```python
from build123d import *

# Parameters (mm, degrees)
F0_R     = 1.375
F0_R_2   = 4.5
F0_W     = 40
F0_H     = 10
F0_W_2   = 10
F0_H_2   = 35
F0_W_3   = 15
F0_H_3   = 2
F0_W_4   = 2
F0_W_5   = 5.5
F0_H_4   = 11.5
F0_R_3   = 1
F1_DEPTH = 3


# Not quite as in the source:
# - a feature names something its author has since deleted; it is built from what else it names


with BuildPart() as f1:
    # F0 (on Top) → F1 (new body)
    with BuildSketch(Plane.XY):
        with BuildLine():
            Line((25, 96.5), (-25, 96.5))
            ThreePointArc((-25, 96.5), (-32.0710678119, 93.5710678119), (-35, 86.5))
            Line((-35, 86.5), (-35, -86.5))
            ThreePointArc((-35, -86.5), (-32.0710678119, -93.5710678119), (-25, -96.5))
            Line((-25, -96.5), (25, -96.5))
            ThreePointArc((25, -96.5), (32.0710678119, -93.5710678119), (35, -86.5))
            Line((35, -86.5), (35, 86.5))
            ThreePointArc((35, 86.5), (32.0710678119, 93.5710678119), (25, 96.5))
        make_face()
        Polygon((-29, -86.5), (-29, -78), (-29, -55), (-29, -46.5), (-25.5, -46.5), (-25.5, -55), (-18.5, -55), (-13, -55), (-10.5, -55), (-10.5, -66.5), (-10.5, -78), (-10.5, -86.5), (-25.5, -86.5), align=None, mode=Mode.SUBTRACT)
        with Locations((-24.5, -8.5)):
            Circle(F0_R, mode=Mode.SUBTRACT)
        Polygon((10.5, -78), (10.5, -66.5), (10.5, -55), (13, -55), (18.5, -55), (24.5, -55), (25.5, -55), (25.5, -46.5), (29, -46.5), (29, -55), (29, -78), (29, -86.5), (25.5, -86.5), (10.5, -86.5), align=None, mode=Mode.SUBTRACT)
        with BuildLine():
            ThreePointArc((25.875, -8.5), (25.4722718241, -9.4722718241), (24.5, -9.875))
            ThreePointArc((24.5, -9.875), (23.5277281759, -7.5277281759), (25.875, -8.5))
        make_face(mode=Mode.SUBTRACT)
        with BuildLine():
            ThreePointArc((26, -30), (25.5980762114, -31.5), (24.5, -32.5980762114))
            ThreePointArc((24.5, -32.5980762114), (23.1822131445, -32.9944612821), (21.8260869565, -32.7607839768))
            ThreePointArc((21.8260869565, -32.7607839768), (0, -52), (-21.8260869565, -32.7607839768))
            ThreePointArc((-21.8260869565, -32.7607839768), (-26, -30), (-21.8260869565, -27.2392160232))
            ThreePointArc((-21.8260869565, -27.2392160232), (-16.3398685927, -15.268785034), (-5, -8.5757147144))
            Line((-5, -8.5757147144), (-5, -5.5))
            Line((-5, -5.5), (-14, -5.5))
            Line((-14, -5.5), (-14, -8.5))
            ThreePointArc((-14, -8.5), (-17, -11.5), (-20, -8.5))
            Line((-20, -8.5), (-20, -5.5))
            Line((-20, -5.5), (-30, -5.5))
            Line((-30, -5.5), (-32, -5.5))
            Line((-32, -5.5), (-32, 6.5))
            Line((-32, 6.5), (-32, 41.5))
            Line((-32, 41.5), (-32, 53.5))
            Line((-32, 53.5), (-30, 53.5))
            Line((-30, 53.5), (-30, 56.5))
            ThreePointArc((-30, 56.5), (-27, 59.5), (-24, 56.5))
            Line((-24, 56.5), (-24, 53.5))
            Line((-24, 53.5), (-20, 53.5))
            Line((-20, 53.5), (20, 53.5))
            Line((20, 53.5), (32, 53.5))
            Line((32, 53.5), (32, 41.5))
            Line((32, 41.5), (32, 6.5))
            Line((32, 6.5), (32, -5.5))
            Line((32, -5.5), (20, -5.5))
            Line((20, -5.5), (5, -5.5))
            Line((5, -5.5), (5, -8.5757147144))
            ThreePointArc((5, -8.5757147144), (16.3398685927, -15.268785034), (21.8260869565, -27.2392160232))
            ThreePointArc((21.8260869565, -27.2392160232), (23.1822131445, -27.0055387179), (24.5, -27.4019237886))
            ThreePointArc((24.5, -27.4019237886), (25.5980762114, -28.5), (26, -30))
        make_face(mode=Mode.SUBTRACT)
        with Locations((0, 81.5)):
            Circle(F0_R_2, mode=Mode.SUBTRACT)
        Polygon((5, 20), (5, 6.5), (20, 6.5), (20, 41.5), (-20, 41.5), (-20, 6.5), (-5, 6.5), (-5, 20), align=None)
        with BuildLine():
            ThreePointArc((-20, -30), (0, -50), (20, -30))
            ThreePointArc((20, -30), (15.8113883008, -17.7525512861), (5, -10.635083269))
            Line((5, -10.635083269), (5, -20))
            Line((5, -20), (-5, -20))
            Line((-5, -20), (-5, -10.635083269))
            ThreePointArc((-5, -10.635083269), (-15.8113883008, -17.7525512861), (-20, -30))
        make_face()
        with Locations((0, 46.5)):
            Rectangle(F0_W, F0_H)
        with Locations((-25, 24)):
            Rectangle(F0_W_2, F0_H_2)
        with Locations((25, 24)):
            Rectangle(F0_W_2, F0_H_2)
        Polygon((-29, -55), (-29, -78), (-25.5, -78), (-18.5, -78), (-18.5, -66.5), (-18.5, -55), (-25.5, -55), align=None)
        with Locations((-24.5, -66.5)):
            Circle(F0_R, mode=Mode.SUBTRACT)
        with BuildLine():
            Line((23.125, -66.5), (18.5, -66.5))
            Line((18.5, -66.5), (18.5, -78))
            Line((18.5, -78), (25.5, -78))
            Line((25.5, -78), (29, -78))
            Line((29, -78), (29, -55))
            Line((29, -55), (25.5, -55))
            Line((25.5, -55), (24.5, -55))
            Line((24.5, -55), (24.5, -65.125))
            ThreePointArc((24.5, -65.125), (25.4722718241, -65.5277281759), (25.875, -66.5))
            ThreePointArc((25.875, -66.5), (24.5, -67.875), (23.125, -66.5))
        make_face()
        with Locations((-12.5, 1.5)):
            Rectangle(F0_W_3, F0_H)
        with Locations((12.5, 1.5)):
            Rectangle(F0_W_3, F0_H)
        Polygon((-18.5, -78), (-25.5, -78), (-25.5, -86.5), (-10.5, -86.5), (-10.5, -78), (-13, -78), align=None)
        Polygon((13, -78), (10.5, -78), (10.5, -86.5), (25.5, -86.5), (25.5, -78), (18.5, -78), align=None)
        with BuildLine():
            ThreePointArc((-21.8260869565, -32.7607839768), (0, -52), (21.8260869565, -32.7607839768))
            ThreePointArc((21.8260869565, -32.7607839768), (20.4978270313, -31.6550318531), (20, -30))
            ThreePointArc((20, -30), (0, -50), (-20, -30))
            ThreePointArc((-20, -30), (-20.4978270313, -31.6550318531), (-21.8260869565, -32.7607839768))
        make_face()
        with Locations((25, 46.5)):
            Rectangle(F0_W_2, F0_H)
        with Locations((-25, 46.5)):
            Rectangle(F0_W_2, F0_H)
        with Locations((-25, 1.5)):
            Rectangle(F0_W_2, F0_H)
        with Locations((25, 1.5)):
            Rectangle(F0_W_2, F0_H)
        with Locations((0, 52.5)):
            Rectangle(F0_W, F0_H_3)
        with Locations((31, 24)):
            Rectangle(F0_W_4, F0_H_2)
        with Locations((-31, 24)):
            Rectangle(F0_W_4, F0_H_2)
        with BuildLine():
            Line((18.5, -55), (18.5, -66.5))
            Line((18.5, -66.5), (23.125, -66.5))
            ThreePointArc((23.125, -66.5), (23.5277281759, -65.5277281759), (24.5, -65.125))
            Line((24.5, -65.125), (24.5, -55))
            Line((24.5, -55), (18.5, -55))
        make_face()
        with Locations((-15.75, -72.25)):
            Rectangle(F0_W_5, F0_H_4)
        with Locations((-15.75, -60.75)):
            Rectangle(F0_W_5, F0_H_4)
        with Locations((15.75, -72.25)):
            Rectangle(F0_W_5, F0_H_4)
        with Locations((15.75, -60.75)):
            Rectangle(F0_W_5, F0_H_4)
        with BuildLine():
            ThreePointArc((-5, -8.5757147144), (-16.3398685927, -15.268785034), (-21.8260869565, -27.2392160232))
            ThreePointArc((-21.8260869565, -27.2392160232), (-20.4978270313, -28.3449681469), (-20, -30))
            ThreePointArc((-20, -30), (-15.8113883008, -17.7525512861), (-5, -10.635083269))
            Line((-5, -10.635083269), (-5, -8.5757147144))
        make_face()
        with BuildLine():
            ThreePointArc((20, -30), (20.4978270313, -28.3449681469), (21.8260869565, -27.2392160232))
            ThreePointArc((21.8260869565, -27.2392160232), (16.3398685927, -15.268785034), (5, -8.5757147144))
            Line((5, -8.5757147144), (5, -10.635083269))
            ThreePointArc((5, -10.635083269), (15.8113883008, -17.7525512861), (20, -30))
        make_face()
        Polygon((30, 41.5), (32, 41.5), (32, 53.5), (20, 53.5), (20, 51.5), (30, 51.5), align=None)
        Polygon((20, -3.5), (20, -5.5), (32, -5.5), (32, 6.5), (30, 6.5), (30, -3.5), align=None)
        Polygon((-14, -5.5), (-5, -5.5), (-5, -3.5), (-20, -3.5), (-20, -5.5), (-17, -5.5), align=None)
        with Locations((12.5, -4.5)):
            Rectangle(F0_W_3, F0_H_3)
        with BuildLine():
            ThreePointArc((-30, 56.5), (-29.1213203519, 54.3786796648), (-27.0000000236, 53.5))
            ThreePointArc((-27.0000000236, 53.5), (-24.8786796648, 54.3786796481), (-24, 56.5))
            ThreePointArc((-24, 56.5), (-27, 59.5), (-30, 56.5))
        make_face()
        with Locations((-27, 56.5)):
            Circle(F0_R_3, mode=Mode.SUBTRACT)
        with BuildLine():
            ThreePointArc((-14, -8.5), (-14.8786796564, -6.3786796564), (-17, -5.5))
            ThreePointArc((-17, -5.5), (-19.1213203436, -6.3786796564), (-20, -8.5))
            ThreePointArc((-20, -8.5), (-17, -11.5), (-14, -8.5))
        make_face()
        with Locations((-17, -8.5)):
            Circle(F0_R_3, mode=Mode.SUBTRACT)
        Polygon((-32, 41.5), (-30, 41.5), (-30, 51.5), (-30, 53.5), (-32, 53.5), align=None)
        Polygon((-30, -5.5), (-30, -3.5), (-30, 6.5), (-32, 6.5), (-32, -5.5), align=None)
        with BuildLine():
            ThreePointArc((-21.8260869565, -27.2392160232), (-26, -30), (-21.8260869565, -32.7607839768))
            ThreePointArc((-21.8260869565, -32.7607839768), (-21.9564786913, -31.3831281496), (-22, -30))
            ThreePointArc((-22, -30), (-21.9564786913, -28.6168718504), (-21.8260869565, -27.2392160232))
        make_face()
        with Locations((-23, -30)):
            Circle(F0_R_3, mode=Mode.SUBTRACT)
        Polygon((-30, 51.5), (-20, 51.5), (-20, 53.5), (-24, 53.5), (-27.0000000236, 53.5), (-30, 53.5), align=None)
        with Locations((-25, -4.5)):
            Rectangle(F0_W_2, F0_H_3)
        with BuildLine():
            ThreePointArc((21.8260869565, -32.7607839768), (23.1822131445, -32.9944612821), (24.5, -32.5980762114))
            Line((24.5, -32.5980762114), (24.5, -27.4019237886))
            ThreePointArc((24.5, -27.4019237886), (23.1822131445, -27.0055387179), (21.8260869565, -27.2392160232))
            ThreePointArc((21.8260869565, -27.2392160232), (21.9564786913, -28.6168718504), (22, -30))
            ThreePointArc((22, -30), (21.9564786913, -31.3831281496), (21.8260869565, -32.7607839768))
        make_face()
        with BuildLine():
            ThreePointArc((24, -30), (23, -31), (22, -30))
            ThreePointArc((22, -30), (23, -29), (24, -30))
        make_face(mode=Mode.SUBTRACT)
        with BuildLine():
            ThreePointArc((-22, -30), (-21.9564786913, -31.3831281496), (-21.8260869565, -32.7607839768))
            ThreePointArc((-21.8260869565, -32.7607839768), (-20.4978270313, -31.6550318531), (-20, -30))
            ThreePointArc((-20, -30), (-20.4978270313, -28.3449681469), (-21.8260869565, -27.2392160232))
            ThreePointArc((-21.8260869565, -27.2392160232), (-21.9564786913, -28.6168718504), (-22, -30))
        make_face()
        with BuildLine():
            ThreePointArc((20, -30), (20.4978270313, -31.6550318531), (21.8260869565, -32.7607839768))
            ThreePointArc((21.8260869565, -32.7607839768), (21.9564786913, -31.3831281496), (22, -30))
            ThreePointArc((22, -30), (21.9564786913, -28.6168718504), (21.8260869565, -27.2392160232))
            ThreePointArc((21.8260869565, -27.2392160232), (20.4978270313, -28.3449681469), (20, -30))
        make_face()
        with BuildLine():
            Line((24.5, -27.4019237886), (24.5, -32.5980762114))
            ThreePointArc((24.5, -32.5980762114), (25.5980762114, -31.5), (26, -30))
            ThreePointArc((26, -30), (25.5980762114, -28.5), (24.5, -27.4019237886))
        make_face()
        with Locations((-23, -30)):
            Circle(F0_R_3)
        with BuildLine():
            ThreePointArc((24, -30), (23, -29), (22, -30))
            ThreePointArc((22, -30), (23, -31), (24, -30))
        make_face()
        with Locations((-27, 56.5)):
            Circle(F0_R_3)
        with Locations((-17, -8.5)):
            Circle(F0_R_3)
        with BuildLine():
            Line((-27.0000000236, 53.5), (-24, 53.5))
            Line((-24, 53.5), (-24, 56.5))
            ThreePointArc((-24, 56.5), (-24.8786796648, 54.3786796481), (-27.0000000236, 53.5))
        make_face()
        with BuildLine():
            Line((-30, 56.5), (-30, 53.5))
            Line((-30, 53.5), (-27.0000000236, 53.5))
            ThreePointArc((-27.0000000236, 53.5), (-29.1213203519, 54.3786796648), (-30, 56.5))
        make_face()
        with BuildLine():
            ThreePointArc((-20, -8.5), (-19.1213203436, -6.3786796564), (-17, -5.5))
            Line((-17, -5.5), (-20, -5.5))
            Line((-20, -5.5), (-20, -8.5))
        make_face()
        with BuildLine():
            Line((-14, -8.5), (-14, -5.5))
            Line((-14, -5.5), (-17, -5.5))
            ThreePointArc((-17, -5.5), (-14.8786796564, -6.3786796564), (-14, -8.5))
        make_face()
    extrude(amount=F1_DEPTH)


solid = f1.part
```
The model under review builds one solid part; all positions refer to its coordinate system, in mm. Give positions to 0.01 mm unless a question says otherwise; leave off trailing zeros. Write each loop counter-clockwise with the first axis right and the second up, starting at its lowest first coordinate (ties: lowest second). Pieces come first, ordered by that corner, then holes. Notation, with made-up numbers: (30.5, 82.5) - (53.5, 82.5) arc R31 ccw to (53.5, 106.5) - close; hole circle Ø5 at (80, 49.5). An arc over 180 degrees is marked (long way). Answer in a Markdown table with one row per item. Add a question column.
1. We need section B-B on y = 81.5. Write out the cut boundary in (x, z), then the cut area to 3 significant figures.
2. We need section C-C on z = 1.35. State how many separate pieces and enclosed holes the cut face has, then the cut area to 3 significant figures.
3. We need section A-A on x = 0. Write out the cut boundary in (y, z), then the cut area to 3 significant figures.
4. Wall thickness on line 1 along Y through (x, z) = (-24.5, 1.8) (3 decimals); line 2 along Y through (x, z) = (0, 0.75); line 3 along X through (y, z) = (-61, 2.7): over which ranges is each line inside the solid? List them lowest first. Write a range as [from, to].
5. Insertion check: P1, Ø0.9, axis at x = 27.5, z = 2, coming from the +Y side. The pin has a flat end and moves straight along its axis. Give the tip position at first contact, or say it passes through.
6. Draft analysis for pull direction X (two halves, no side actions). For faces 1 (the flat face through (-8, 1, 0)), 2 (the cylindrical face through (31.99, -93.65, 1.48)), 3 (the cylindrical face through (-0.59, 85.96, 1.48)), state which applies: +X half, -X half, draft (parallel to the pull), parting line (faces both ways), or undercut.
Ans:
| question | item | result |
|---|---|---|
| 1 | outline | (-35, 0) - (-4.5, 0) - (-4.5, 3) - (-35, 3) - close; (4.5, 0) - (35, 0) - (35, 3) - (4.5, 3) - close |
| 1 | area | 183 mm^2 |
| 2 | separate pieces | 1 |
| 2 | enclosed holes | 12 |
| 2 | area | 12,700 mm^2 |
| 3 | outline | (-96.5, 0) - (-20, 0) - (-20, 3) - (-96.5, 3) - close; (20, 0) - (77, 0) - (77, 3) - (20, 3) - close; (86, 0) - (96.5, 0) - (96.5, 3) - (86, 3) - close |
| 3 | area | 432 mm^2 |
| 4 | line 1 | y = [-96.5, -67.875], [-65.125, -9.875], [-7.125, 96.5] |
| 4 | line 2 | y = [-96.5, -20], [20, 77], [86, 96.5] |
| 4 | line 3 | x = [-35, -13], [-10.5, 10.5], [13, 35] |
| 5 | P1 | stops at y = 96.29 |
| 6 | face 1 | draft |
| 6 | face 2 | +X half |
| 6 | face 3 | undercut |
